Geometry check sheet. Reference: the model listing, model coordinates, mm. Give positions to 0.01 mm unless a question says otherwise; leave off trailing zeros. Order: outer loops, then holes, each group sorted by start corner. A loop starts at its lowest first (then second) coordinate and runs counter-clockwise, first axis right, second up.
Autodesk Inventor part; units mm, degrees
ref_plane "YZ Plane" through (0, 0, 0) normal (1, 0, 0) x (0, 1, 0)
ref_plane "XZ Plane" through (0, 0, 0) normal (0, 1, 0) x (-1, 0, 0)
ref_plane "XY Plane" through (0, 0, 0) normal (0, 0, 1) x (1, 0, 0)
sketch "Sketch1" plane through (0, 0, 0) normal (0, 0, 1) x (1, 0, 0)
  line L0 (0, 0) -> (236, 0)
  line L1 (236, 0) -> (236, 40)
  line L2 (236, 40) -> (0, 40)
  line L3 (0, 40) -> (0, 0)
  dimension "d0" = 236
  dimension "d1" = 40
extrude "Extrusion1" add sketch "Sketch1" along normal blind 5
sketch "Sketch2" plane through (0, 0, 5) normal (0, 0, 1) x (1, 0, 0)
  line L0 (236, 40) -> (0, 40)
  line L1 (0, 0) -> (236, 0)
  line L2 (0, 40) -> (0, 0)
  point P0 (43, 30)
  point P1 (43, 10)
  dimension "d4" = 10
  dimension "d6" = 43
  dimension "d40" = 20
  dimension "d41" = 10
hole "Hole1" at (43, 30, 5) at (43, 10, 5) direction (0, 0, -1) diameter 4.5 end through all
pattern_linear "Rectangular Pattern1" count 4 spacing 50 along (1, 0, 0) of "Hole1"
sketch "Sketch3" plane through (0, 0, 5) normal (0, 0, 1) x (1, 0, 0)
  line L0 (236, 40) -> (0, 40)
  line L1 (0, 40) -> (0, 0)
  line L2 (236, 0) -> (236, 40)
  point P0 (68.4243, 20)
  point P1 (167.5757, 7)
  dimension "d17" = 100
  dimension "d18" = 20
  dimension "d19" = 13
  dimension "d20" = 68.4243
  dimension "d21" = 68.4243
hole "Hole2" at (68.4243, 20, 5) at (167.5757, 7, 5) direction (0, 0, -1) diameter 4.5 end through all
sketch "Sketch4" plane through (0, 0, 5) normal (0, 0, 1) x (1, 0, 0)
  line L0 (236, 40) -> (0, 40)
  line L1 (0, 0) -> (236, 0)
  line L2 (0, 40) -> (0, 0)
  line L3 (236, 0) -> (236, 40)
  point P0 (12.5, 32.5)
  point P1 (12.5, 7.5)
  point P2 (223.5, 32.5)
  point P3 (223.5, 7.5)
  dimension "d29" = 7.5
  dimension "d30" = 7.5
  dimension "d31" = 12.5
  dimension "d32" = 12.5
hole "Hole3" at (12.5, 32.5, 5) at (12.5, 7.5, 5) at (223.5, 32.5, 5) at (223.5, 7.5, 5) direction (0, 0, -1) diameter 4.5 end through all
sketch "Sketch5" plane through (0, 0, 5) normal (0, 0, 1) x (1, 0, 0)
  line L0 (236, 40) -> (0, 40)
  line L1 (236, 0) -> (236, 40)
  line L2 (0, 40) -> (0, 0)
  point P0 (25, 35)
  point P1 (211, 35)
  dimension "d42" = 5
  dimension "d51" = 25
  dimension "d52" = 25
hole "Hole4" at (25, 35, 5) at (211, 35, 5) direction (0, 0, -1) diameter 3 end through all
properties part number "Top_Slider Piece 1_4 Lanes" material "Wood (Oak)"
Item 1: Scan lines: L1, parallel to X at y = 30, z = 0.95; L2, parallel to Y at x = 223.5, z = 3.5; L3, parallel to X at y = 7.5, z = 2.7. Record each from-to range of solid material in increasing order.
Reported:
L1: x = 0 to 40.75, 45.25 to 90.75, 95.25 to 140.75, 145.25 to 190.75, 195.25 to 236
L2: y = 0 to 5.25, 9.75 to 30.25, 34.75 to 40
L3: x = 0 to 10.25, 14.75 to 165.38, 169.77 to 221.25, 225.75 to 236
Item 2: Sectioned sample at A-A (x = 143). Enter the section's corners in (y, z).
Reported:
outline: (0, 0) - (7.75, 0) - (7.75, 5) - (0, 5) - close; (12.25, 0) - (27.75, 0) - (27.75, 5) - (12.25, 5) - close; (32.25, 0) - (40, 0) - (40, 5) - (32.25, 5) - close
Item 3: Sectioned sample at B-B (z = 4.15). Give the number of separate pieces and of enclosed holes in the cut face, and give its area (3 significant figures).
Reported:
separate pieces: 1
enclosed holes: 16
area: 9,200 mm2
Item 4: Draft check along X on faces 1 (the cylindrical face through (145.196, 10.488, 2.465)), 2 (the flat face through (236, 20, 2)), 3 (the flat face through (0, 20, 2)). Enter one of: released by +X, released by -X, zero draft, split by the parting line, or undercut.
Reported:
face 1: undercut
face 2: released by +X
face 3: released by -X
